```python
from build123d import *

# Parameters (mm, degrees)
IZIM2_W                     = 15
IZIM2_H                     = 9.6
Y_KSEKLIK_EKSTR_ZYON1_DEPTH = 2.4
IZIM3_W                     = 6
IZIM3_H                     = 6
Y_KSEKLIK_EKSTR_ZYON2_DEPTH = 3.5
IZIM4_R                     = 1.75
Y_KSEKLIK_EKSTR_ZYON3_DEPTH = 2.5


with BuildPart() as part:
    # Çizim2 → Yükseklik-Ekstrüzyon1 (new body)
    with BuildSketch(Plane.XY):
        Rectangle(IZIM2_W, IZIM2_H)
    extrude(amount=Y_KSEKLIK_EKSTR_ZYON1_DEPTH)

    # Çizim3 → Yükseklik-Ekstrüzyon2 (add)
    with BuildSketch(Plane.XY.offset(2.4)):
        Rectangle(IZIM3_W, IZIM3_H)
    extrude(amount=Y_KSEKLIK_EKSTR_ZYON2_DEPTH)

    # Çizim4 → Yükseklik-Ekstrüzyon3 (add)
    with BuildSketch(Plane.XY.offset(5.9)):
        Circle(IZIM4_R)
    extrude(amount=Y_KSEKLIK_EKSTR_ZYON3_DEPTH)


solid = part.part
```
Geometry: final body of the model. Coordinates: model frame, mm. A direction names the side the tool comes from. Give positions to 0.01 mm unless a question says otherwise; leave off trailing zeros. Order: outer loops, then holes, each group sorted by start corner. A loop starts at its lowest first (then second) coordinate and runs counter-clockwise, first axis right, second up. Notation, with made-up numbers: (41, -3.75) -> (74, -3.75) arc R18 ccw to (74, 23.25) -> close; hole circle Ø10 at (12, 32.5). An arc over 180 degrees is marked (long way). Write each question's results on one line, items separated by ' | '. Start each with the question number.
1) Section A-A (y = 0). Return loops of the section in (x, z).
2) Line query: line 1 (Y direction, x = -2, z = 4); line 2 (Z direction, x = -6.25, y = -1.5). Output: solid intervals per line, ascending. Write a range as from..to.
3) Section D-D (y = 2). Return loops of the section in (x, z), then the cut area to 3 significant figures.
4) Set-up query: faces 1 (the flat face through (3, 0, 4)), 2 (the flat face through (1.3, 1.4, 5.9)), 3 (the flat face through (0, 3, 4)), 4 (the flat face through (0, -3, 4)). Return all of +Z, -Z, +X, -X, +Y, -Y with unobstructed straight access to the full face (end or side cutting, diameter ignored); none if empty.
5) Section B-B (x = 2.5). Return loops of the section in (y, z), then the cut area to 3 significant figures.
6) First-contact query: pin 1 (1.8 mm diameter, centred on y = 1, z = 4.5, fed in from -X); pin 2 (1 mm diameter, centred on x = 1.5, z = 4, fed in from +Y); pin 3 (1 mm diameter, centred on x = 1, z = 3.5, fed in from -Y). Flat tips, straight axial feed; report the tip coordinate or a pass-through.
7) Section C-C (z = 2.75). Return loops of the section in (x, y).
Calculated:
1) outline: (-7.5, 0) -> (7.5, 0) -> (7.5, 2.4) -> (3, 2.4) -> (3, 5.9) -> (1.75, 5.9) -> (1.75, 8.4) -> (-1.75, 8.4) -> (-1.75, 5.9) -> (-3, 5.9) -> (-3, 2.4) -> (-7.5, 2.4) -> close
2) line 1: -3..3 | line 2: 0..2.4
3) outline: (-7.5, 0) -> (7.5, 0) -> (7.5, 2.4) -> (3, 2.4) -> (3, 5.9) -> (-3, 5.9) -> (-3, 2.4) -> (-7.5, 2.4) -> close | area: 57.0 mm2
4) face 1: +Z, +X, +Y, -Y | face 2: +Z | face 3: +Z, +X, -X, +Y | face 4: +Z, +X, -X, -Y
5) outline: (-4.8, 0) -> (4.8, 0) -> (4.8, 2.4) -> (3, 2.4) -> (3, 5.9) -> (-3, 5.9) -> (-3, 2.4) -> (-4.8, 2.4) -> close | area: 44.0 mm2
6) pin 1: x = -3 | pin 2: y = 3 | pin 3: y = -3
7) outline: (-3, -3) -> (3, -3) -> (3, 3) -> (-3, 3) -> close
